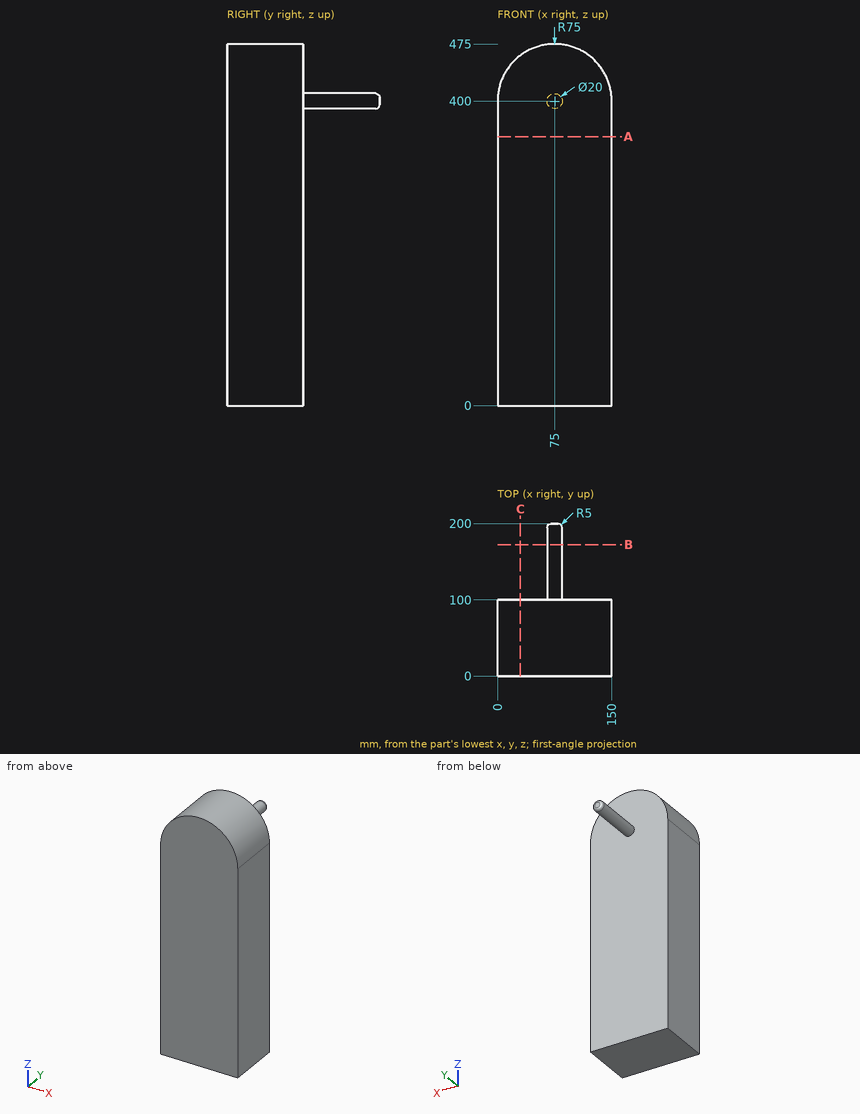
For this review, use the dimensioned drawing (mm, ordinates from the lowest corner) and the shaded views. Coordinates: 2 decimals unless noted, no trailing zeros. Loops run counter-clockwise (first coordinate to the right, second up) from the corner with the lowest first, then second, coordinate; pieces in that order, holes last.
1. Add section A-A, the plane z = 353.5. Give the boundary of the cut face in (x, y).
2. Add section B-B, the plane y = 172.5. Give the boundary of the cut face in (x, z).
3. Insertion check: P1, Ø3, axis at x = 134.5, y = 48.5, coming from the +Z side; P2, Ø8, axis at x = 22, z = 285, coming from the +Y side. Each pin has a flat end and moves straight along its axis. Give the tip position at first contact, or say it passes through.
4. Add section C-C, the plane x = 30. Give the boundary of the cut face in (y, z), then the cut area to 3 significant figures.
5. For line 1 (Y direction, x = 70, z = 41); line 2 (Z direction, x = 47, y = 66.5); line 3 (Z direction, x = 137.5, y = 33), list the stretches that pass through material, from the lowest coordinate up.
Result:
1. outline: (0, 0) - (150, 0) - (150, 100) - (0, 100) - close
2. outline: circle Ø20 at (75, 400)
3. P1: stops at z = 447.55
3. P2: stops at y = 100
4. outline: (0, 0) - (100, 0) - (100, 460) - (0, 460) - close
4. area: 46,000 mm2
5. line 1: y = 0 to 100
5. line 2: z = 0 to 469.58
5. line 3: z = 0 to 441.46
